Here's the drawing with two shaded views (mm, measured from the low corner). I have some questions. A direction names the side the tool comes from. Coordinates: 2 decimals unless noted, no trailing zeros. Write each loop counter-clockwise with the first axis right and the second up, starting at its lowest first coordinate (ties: lowest second). Pieces come first, ordered by that corner, then holes. Notation, with made-up numbers: (-35.5, 52) - (4.5, 52) arc R22 ccw to (4.5, 76) - close; hole circle Ø7 at (82, 5.5). An arc over 180 degrees is marked (long way). Answer in a Markdown table with one row per item. Add a question column.
Item 1: We'd pull the mould along Y, two halves only. Please class the marked faces 4, 5, 6 and 7: +Y half, -Y half, draft (parallel to the pull), parting line (faces both ways), or undercut.
Item 2: Which directions (+Z, -Z, +X, -X, +Y, -Y) give clear straight access to the entire face, cutting with the end or side of a thin tool? Please do the marked faces 1, 2 and 3.
Item 3: Imagine slicing it at C-C (x = 40). Please give me the cut outline in (y, z).
Item 4: I'm going to push flat-ended pins straight in: pin 1 (3 mm diameter, centred on x = 28, y = 89, fed in from -Z); pin 2 (10 mm diameter, centred on x = 39.5, y = 103, fed in from -Z); pin 3 (10 mm diameter, centred on x = 10, y = 105, fed in from -Z); pin 4 (4 mm diameter, centred on x = 20, z = 14.5, fed in from +Y). Where does each tip first touch, or does it pass through?
Item 5: Imagine slicing it at D-D (x = 22). Please give me the cut outline in (y, z).
Item 6: Imagine slicing it at B-B (y = 15). Please give me the cut outline in (x, z), plus the area to 3 significant figures.
Item 7: Imagine slicing it at A-A (z = 35). Please give me the cut outline in (x, y), plus the area to 3 significant figures.
Item 8: If I drill on probe 1 along X at (y, z) = (108.5, 34); probe 2 along Y at (x, z) = (10, 26.25); probe 3 along Y at (x, z) = (40, 24.25), over which ranges is the centre line in solid material (lowest first)? Write a range as from..to.
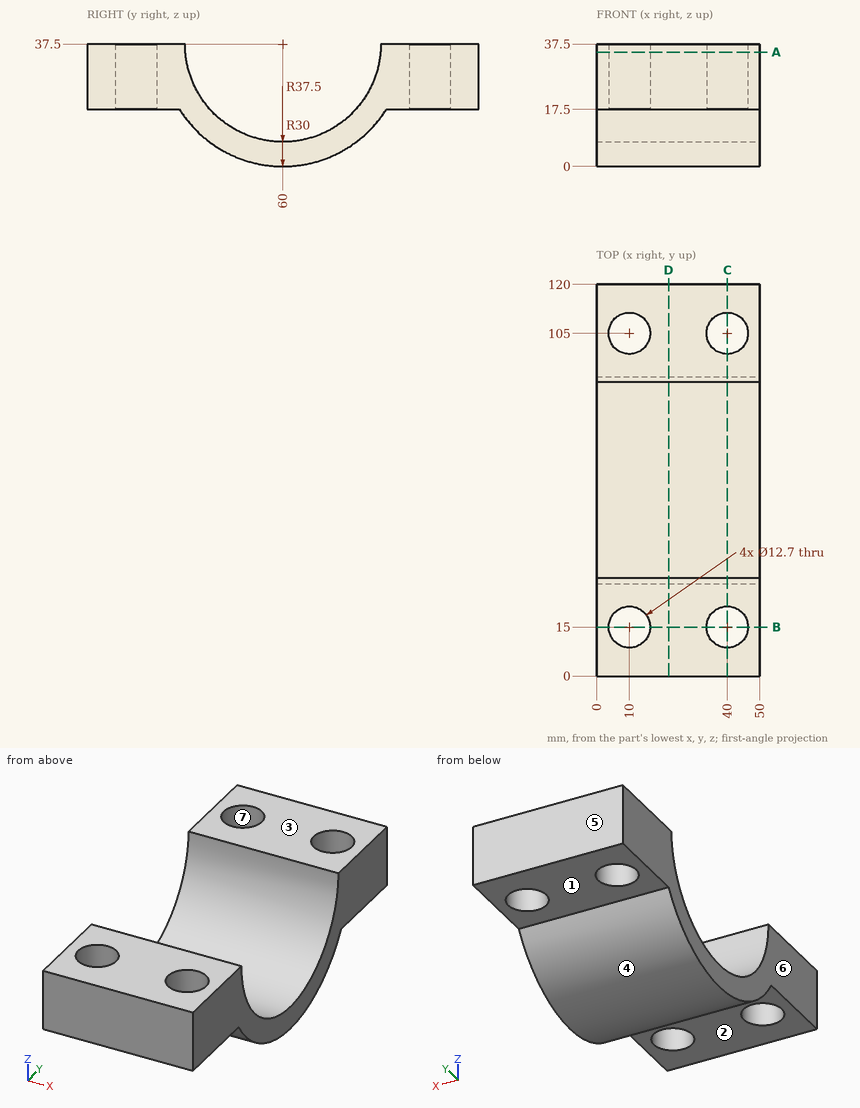
Here are the results:
| question | item | result |
|---|---|---|
| 1 | face 4 | parting line |
| 1 | face 5 | +Y half |
| 1 | face 6 | draft |
| 1 | face 7 | undercut |
| 2 | face 1 | -Z, +X, -X, +Y |
| 2 | face 2 | -Z, +X, -X, -Y |
| 2 | face 3 | +Z, +X, -X, +Y, -Y |
| 3 | outline | (0, 17.5) - (8.65, 17.5) - (8.65, 37.5) - (0, 37.5) - close; (21.35, 17.5) - (28.28, 17.5) arc R37.5 ccw to (91.72, 17.5) - (98.65, 17.5) - (98.65, 37.5) - (90, 37.5) arc R30 cw to (30, 37.5) - (21.35, 37.5) - close; (111.35, 17.5) - (120, 17.5) - (120, 37.5) - (111.35, 37.5) - close |
| 4 | pin 1 | stops at z = 12 |
| 4 | pin 2 | stops at z = 17.5 |
| 4 | pin 3 | passes through |
| 4 | pin 4 | stops at y = 91.07 |
| 5 | outline | (0, 17.5) - (28.28, 17.5) arc R37.5 ccw to (91.72, 17.5) - (120, 17.5) - (120, 37.5) - (90, 37.5) arc R30 cw to (30, 37.5) - (0, 37.5) - close |
| 6 | outline | (0, 17.5) - (3.65, 17.5) - (3.65, 37.5) - (0, 37.5) - close; (16.35, 17.5) - (33.65, 17.5) - (33.65, 37.5) - (16.35, 37.5) - close; (46.35, 17.5) - (50, 17.5) - (50, 37.5) - (46.35, 37.5) - close |
| 6 | area | 492 mm2 |
| 7 | outline | (0, 0) - (50, 0) - (50, 30.1) - (0, 30.1) - close; (0, 89.9) - (50, 89.9) - (50, 120) - (0, 120) - close; hole circle Ø12.7 at (10, 15); hole circle Ø12.7 at (10, 105); hole circle Ø12.7 at (40, 15); hole circle Ø12.7 at (40, 105) |
| 7 | area | 2,500 mm2 |
| 8 | probe 1 | x = 0..4.7, 15.3..34.7, 45.3..50 |
| 8 | probe 2 | y = 0..8.65, 21.35..32.19, 87.81..98.65, 111.35..120 |
| 8 | probe 3 | y = 0..8.65, 21.35..33.08, 86.92..98.65, 111.35..120 |
